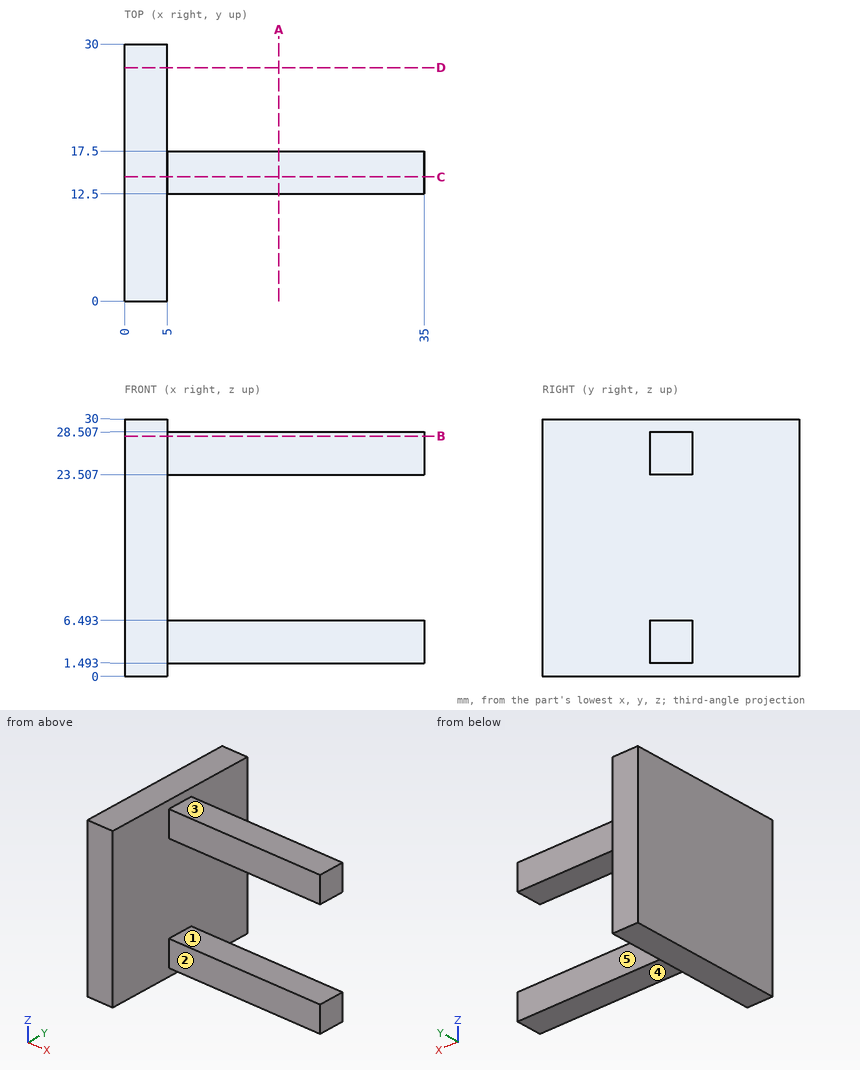
Design review of the part shown in the three views and the two pictorial views. Dimensions are in mm from the part's minimum x, y and z. A direction names the side the tool comes from. Give positions to 0.01 mm unless a question says otherwise; leave off trailing zeros. Loops run counter-clockwise (first coordinate to the right, second up) from the corner with the lowest first, then second, coordinate; pieces in that order, holes last. Notation, with made-up numbers: (-29, 50) - (-11, 50) arc R30 cw to (-11, 82) - close; hole circle Ø11 at (33.5, -22.5). An arc over 180 degrees is marked (long way). Use CSV: the item, a comma, the result in double quotes. Start each with the question number.
1. Machinability: for the marked faces 1, 2, 3, 4 and 5, which of the approach directions +Z, -Z, +X, -X, +Y, -Y give a long, thin tool a straight path to every point of the face, cutting with its end or side? Answer none if there is none.
2. Wall thickness on L1, parallel to Z at x = 18.5, y = 12.75; L2, parallel to Y at x = 16, z = 25.5; L3, parallel to X at y = 25, z = 15: over which ranges is each line inside the solid? List them lowest first.
3. Add section C-C (y = 14.5). State the section outline as (x, z) points, plus the area to 3 significant figures.
4. Add section B-B (z = 28). State the section outline as (x, y) points, plus the area to 3 significant figures.
5. Insertion check: P1, Ø2.5, axis at x = 13, y = 14, coming from the +Z side; P2, Ø4, axis at x = 17.5, y = 15, coming from the -Z side; P3, Ø4, axis at x = 21, z = 25.5, coming from the -Y side. Each pin has a flat end and moves straight along its axis. Give the tip position at first contact, or say it passes through.
6. Add section D-D (y = 27.25). State the section outline as (x, z) points.
7. Add section A-A (x = 18). State the section outline as (y, z) points.
Results found:
1,face 1,"+X, +Y, -Y"
1,face 2,"+Z, -Z, +X, -Y"
1,face 3,"+Z, +X, +Y, -Y"
1,face 4,"-Z, +X, +Y, -Y"
1,face 5,"+Z, -Z, +X, +Y"
2,L1,"z = 1.49 to 6.49, 23.51 to 28.51"
2,L2,"y = 12.5 to 17.5"
2,L3,"x = 0 to 5"
3,outline,"(0, 0) - (5, 0) - (5, 1.49) - (35, 1.49) - (35, 6.49) - (5, 6.49) - (5, 23.51) - (35, 23.51) - (35, 28.51) - (5, 28.51) - (5, 30) - (0, 30) - close"
3,area,"450 mm²"
4,outline,"(0, 0) - (5, 0) - (5, 12.5) - (35, 12.5) - (35, 17.5) - (5, 17.5) - (5, 30) - (0, 30) - close"
4,area,"300 mm²"
5,P1,"stops at z = 28.51"
5,P2,"stops at z = 1.49"
5,P3,"stops at y = 12.5"
6,outline,"(0, 0) - (5, 0) - (5, 30) - (0, 30) - close"
7,outline,"(12.5, 1.49) - (17.5, 1.49) - (17.5, 6.49) - (12.5, 6.49) - close; (12.5, 23.51) - (17.5, 23.51) - (17.5, 28.51) - (12.5, 28.51) - close"
